```python
from build123d import *

# Parameters (mm, degrees)
SKETCH1_W               = 15.577947364
SKETCH1_H               = 15.577947364
BOSS_EXTRUDE2_DEPTH     = 10
CUT_EXTRUDE1_DEPTH      = 15.877372821
CUT_EXTRUDE1_DEPTH_BACK = 15.877372821
SKETCH2_R               = 2.35
FILLET3_SIZE            = 3.3
CUT_EXTRUDE2_DEPTH      = 21.083340288
CUT_EXTRUDE2_DEPTH_BACK = 21.083340288
SKETCH9_W               = 17.356055064
SKETCH9_H               = 10.947578027


with BuildPart() as part:
    # Sketch1 → Boss-Extrude2 (new body)
    with BuildSketch(Plane(origin=(0, 0, 0), x_dir=(1, 0, 0), z_dir=(0, 1, 0))):
        Rectangle(SKETCH1_W, SKETCH1_H)
    extrude(amount=BOSS_EXTRUDE2_DEPTH)

    # Sketch2 → Cut-Extrude1 (cut, two sides: drawn at the far end of the back side and taken through both)
    with BuildSketch(Plane(origin=(0, 10, 0), x_dir=(1, 0, 0), z_dir=(0, 1, 0)).offset(-CUT_EXTRUDE1_DEPTH_BACK)):
        with Locations(Location((0, 0, 0), (0, 0, 270))):
            Circle(SKETCH2_R)
    extrude(amount=CUT_EXTRUDE1_DEPTH + CUT_EXTRUDE1_DEPTH_BACK, mode=Mode.SUBTRACT)

    # Fillet3
    # a fillet whose section is not a circle: 3.3 mm, written as the material it takes off along each edge
    with BuildSketch(Plane(origin=(0, 10, 0), x_dir=(0, 0, 1), z_dir=(-1, 0, 0))) as fillet3_piece_1:
        with BuildLine():
            Bezier((2.35 + FILLET3_SIZE, 0), (2.35, 0), (2.35, -FILLET3_SIZE), weights=[1, 0.016667517, 1])
            Line((2.35, -FILLET3_SIZE), (2.35, 0))
            Line((2.35, 0), (2.35 + FILLET3_SIZE, 0))
        make_face()
    revolve(axis=Axis((0, 10, 0), (0, 1, 0)), mode=Mode.SUBTRACT)

    # Sketch9 → Cut-Extrude2 (cut, two sides: drawn at the far end of the back side and taken through both)
    with BuildSketch(Plane.ZY.offset(7.788973682).offset(-CUT_EXTRUDE2_DEPTH_BACK)):
        with Locations((-0.203270831, -0.297866067)):
            Rectangle(SKETCH9_W, SKETCH9_H)
    extrude(amount=CUT_EXTRUDE2_DEPTH + CUT_EXTRUDE2_DEPTH_BACK, mode=Mode.SUBTRACT)


solid = part.part
```
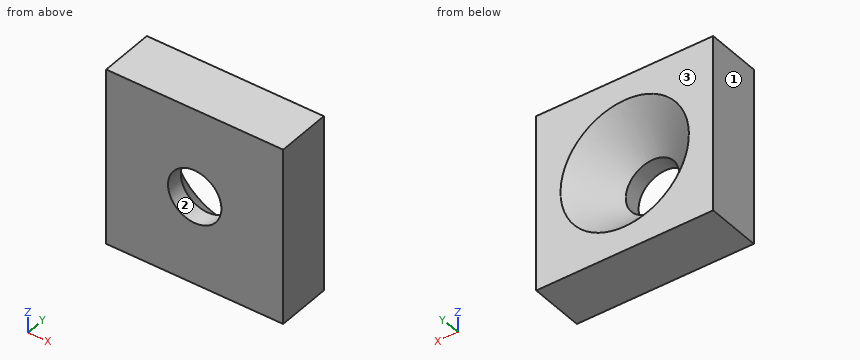
Geometry: final body of the model. Coordinates: model frame, mm. Face numbers are marked on the shaded views. Coordinates: 2 decimals unless noted, no trailing zeros. Answer in a Markdown table with one row per item.
Item 1: Contact query for flat-ended pins moving along their axis: P1, Ø3, axis at x = 4, z = -0.5, coming from the +Y side; P2, Ø4, axis at x = 0, z = 0, coming from the -Y side. Output: stop coordinate, or through.
Return value:
| item | result |
|---|---|
| P1 | stops at y = 9.9 |
| P2 | passes through |
Item 2: Draft query along X for the marked faces 1, 2 and 3. Return one class per face: released by +X, released by -X, zero draft, split by the parting line, or undercut.
Return value:
| item | result |
|---|---|
| face 1 | released by -X |
| face 2 | undercut |
| face 3 | zero draft |
Item 3: Ray query, L1, parallel to X at y = 5.5, z = 0; L2, parallel to X at y = 8.6, z = -3. Return the intervals inside material, ascending.
Return value:
| item | result |
|---|---|
| L1 | x = -7.79 to -2.35, 2.35 to 7.79 |
| L2 | x = -7.79 to -2.93, 2.93 to 7.79 |
